Design review of the part shown in the three views and the two pictorial views. Dimensions are in mm from the part's minimum x, y and z. Give positions to 0.01 mm unless a question says otherwise; leave off trailing zeros. Order: outer loops, then holes, each group sorted by start corner. A loop starts at its lowest first (then second) coordinate and runs counter-clockwise, first axis right, second up. Notation, with made-up numbers: (-38, -29) -> (-1, -29) arc R21 cw to (-1, -9) -> close; hole circle Ø11 at (7.25, 82). An arc over 180 degrees is marked (long way). Use one line per item in the form item = value.
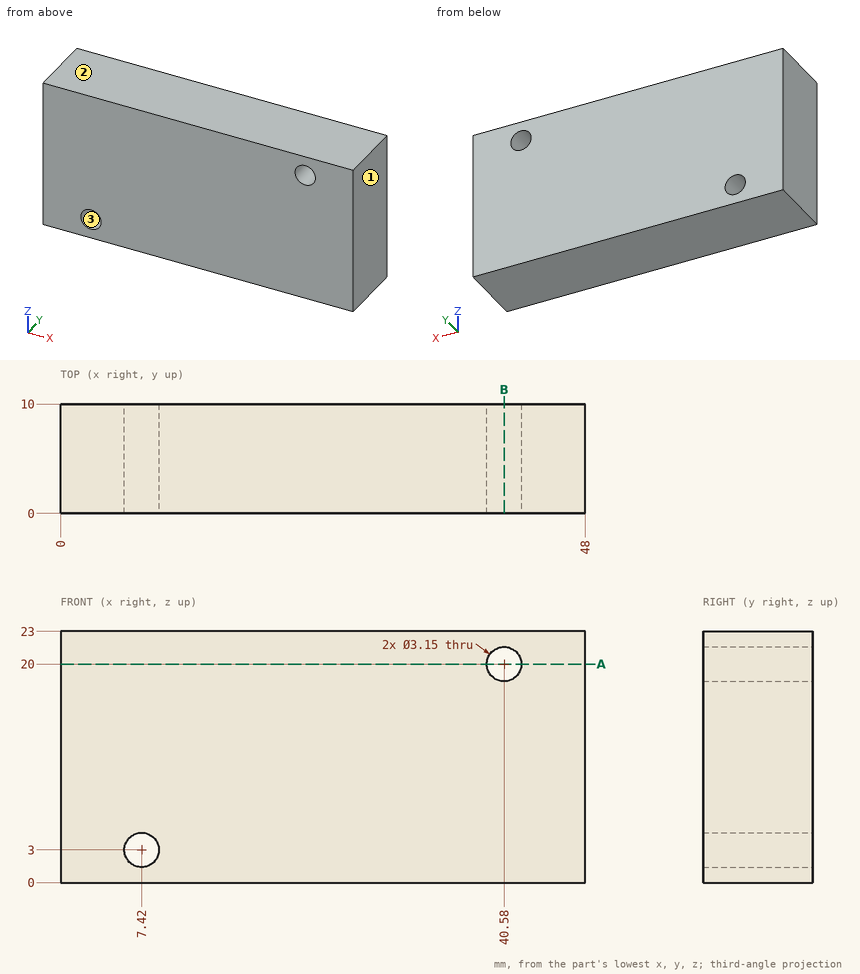
1. Add section B-B on x = 40.58. Give the boundary of the cut face in (y, z) (3 decimals).
Values:
outline = (0, 0) -> (10, 0) -> (10, 18.425) -> (0, 18.425) -> close; (0, 21.575) -> (10, 21.575) -> (10, 23) -> (0, 23) -> close
2. For L1, parallel to X at y = 7, z = 3 (3 decimals); L2, parallel to Z at x = 40.58, y = 2.5 (3 decimals); L3, parallel to X at y = 7.5, z = 20 (3 decimals), list the stretches that pass through material, from the lowest coordinate up.
Values:
L1 = 0 to 5.845, 8.995 to 48
L2 = 0 to 18.425, 21.575 to 23
L3 = 0 to 39.005, 42.155 to 48
3. The part is to be moulded in two halves that separate along Z. For the marked faces 1, 2 and 3, say which applies: +Z half, -Z half, draft (parallel to the pull), parting line (faces both ways), or undercut.
Values:
face_1 = draft
face_2 = +Z half
face_3 = undercut
4. Add section A-A on z = 20. Give the boundary of the cut face in (x, y) (3 decimals).
Values:
outline = (0, 0) -> (39.005, 0) -> (39.005, 10) -> (0, 10) -> close; (42.155, 0) -> (48, 0) -> (48, 10) -> (42.155, 10) -> close
